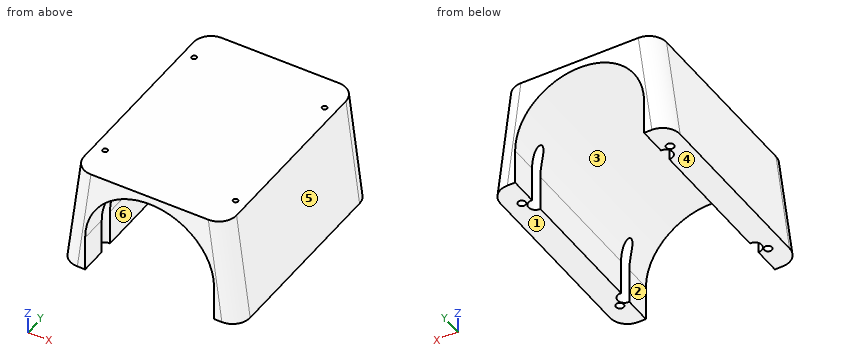
```python
from build123d import *

# Parameters (mm, degrees)
POCKET_DEPTH    = 110.201
SKETCH003_R     = 1.95
POCKET001_DEPTH = 30
SKETCH004_R     = 1.25
POCKET002_DEPTH = 55.001
SKETCH005_R     = 3.5
POCKET003_DEPTH = 50


with BuildPart() as part:
    # Sketch → Loft section 0
    with BuildSketch(Plane.XY):
        with BuildLine():
            Line((-37, 55.1), (37, 55.1))
            ThreePointArc((46, 46.1), (43.363961, 52.463961), (37, 55.1))
            Line((46, 46.1), (46, -46.1))
            ThreePointArc((37, -55.1), (43.363961, -52.463961), (46, -46.1))
            Line((37, -55.1), (-37, -55.1))
            ThreePointArc((-46, -46.1), (-43.363961, -52.463961), (-37, -55.1))
            Line((-46, -46.1), (-46, 46.1))
            ThreePointArc((-37, 55.1), (-43.363961, 52.463961), (-46, 46.1))
        make_face()
    # Sketch001 → Loft section 1
    with BuildSketch(Plane.XY.offset(55)):
        with BuildLine():
            Line((-30.05, 55.1), (30.05, 55.1))
            ThreePointArc((39.05, 46.1), (36.413961, 52.463961), (30.05, 55.1))
            Line((39.05, 46.1), (39.05, -46.1))
            ThreePointArc((30.05, -55.1), (36.413961, -52.463961), (39.05, -46.1))
            Line((30.05, -55.1), (-30.05, -55.1))
            ThreePointArc((-39.05, -46.1), (-36.413961, -52.463961), (-30.05, -55.1))
            Line((-39.05, -46.1), (-39.05, 46.1))
            ThreePointArc((-30.05, 55.1), (-36.413961, 52.463961), (-39.05, 46.1))
        make_face()
    loft()

    # Sketch002 (on Face5 of BaseFeature) → Pocket (cut, through all)
    with BuildSketch(Plane.XZ.offset(55.1)):
        with BuildLine():
            Line((33, 18), (33, 0))
            Line((33, 0), (-33, 0))
            Line((-33, 0), (-33, 18))
            ThreePointArc((33, 18), (0, 51), (-33, 18))
        make_face()
    extrude(amount=-POCKET_DEPTH, mode=Mode.SUBTRACT)

    # Sketch003 (on Face5 of Pocket) → Pocket001 (cut)
    with BuildSketch(Plane(origin=(0, 0, 0), x_dir=(1, 0, 0), z_dir=(0, 0, -1))):
        with Locations((-37.95, 41.3)):
            Circle(SKETCH003_R)
        with Locations((-37.95, -41.3)):
            Circle(SKETCH003_R)
        with Locations((37.95, -41.3)):
            Circle(SKETCH003_R)
        with Locations((37.95, 41.3)):
            Circle(SKETCH003_R)
    extrude(amount=-POCKET001_DEPTH, mode=Mode.SUBTRACT)

    # Sketch004 (on Face3 of Pocket001) → Pocket002 (cut, through all)
    with BuildSketch(Plane.XY.offset(55)):
        with Locations((-33.4, 37.35)):
            Circle(SKETCH004_R)
        with Locations((33.4, 37.35)):
            Circle(SKETCH004_R)
        with Locations((33.4, -37.65)):
            Circle(SKETCH004_R)
        with Locations((-33.4, -37.65)):
            Circle(SKETCH004_R)
    extrude(amount=-POCKET002_DEPTH, mode=Mode.SUBTRACT)

    # Sketch005 (on Face9 of Pocket002) → Pocket003 (cut)
    with BuildSketch(Plane(origin=(0, 0, 0), x_dir=(1, 0, 0), z_dir=(0, 0, -1))):
        with Locations((-33.4, -37.35)):
            Circle(SKETCH005_R)
        with Locations((33.4, -37.35)):
            Circle(SKETCH005_R)
        with Locations((-33.4, 37.65)):
            Circle(SKETCH005_R)
        with Locations((33.4, 37.65)):
            Circle(SKETCH005_R)
    extrude(amount=-POCKET003_DEPTH, mode=Mode.SUBTRACT)


solid = part.part
```
Verification items for the finished model (mm, model axes). Face numbers are marked on the shaded views. A direction names the side the tool comes from. Round coordinates to 2 decimals unless told otherwise and drop trailing zeros. Write each loop counter-clockwise with the first axis right and the second up, starting at its lowest first coordinate (ties: lowest second). Pieces come first, ordered by that corner, then holes. Notation, with made-up numbers: (43, 1.5) - (53, 1.5) arc R24 cw to (53, 28.5) - close; hole circle Ø3 at (19.25, 73.25). An arc over 180 degrees is marked (long way). Answer as a JSON object with one key per item and string values. Group by question number.
Q1. Section check B-B, the plane z = 37. Give the number of separate pieces and of enclosed holes in the cut face, plus the area to 3 significant figures.
Q2. Mould release check, pull along X, two halves, no side actions. Record for the marked faces 3, 4, 5 and 6: released by +X, released by -X, zero draft, split by the parting line, or undercut.
Q3. Go/stop test with flat-tipped pins: pin 1 Ø1.5 at (x, z) = (28.5, 31) entering from +Y; pin 2 Ø5 at (x, y) = (37.95, 41.3) entering from -Z; pin 3 Ø1 at (y, z) = (-32.5, 21.5) entering from -X; pin 4 Ø2.5 at (x, y) = (37.95, -41.3) entering from -Z. Record where each tip stops, or that it passes through.
Q4. Thickness scan on line 1 (Y direction, x = 33, z = 34.5); line 2 (X direction, y = -41.3, z = 21.5); line 3 (Y direction, x = -37, z = 10). Record the ranges inside material, lowest first.
Q5. Section check A-A, the plane y = -29. Enter the section's corners in (x, z), plus the area to 3 significant figures.
Q6. Tool access check on the marked faces 1 and 2. Record the directions out of +Z, -Z, +X, -X, +Y, -Y that give a thin tool (end or side, any length) a straight path to the whole face; none if there is none.
Found:
{
 "1": {"separate pieces": "2", "enclosed holes": "4", "area": "2,940 mm^2"},
 "2": {"face 3": "undercut", "face 4": "zero draft", "face 5": "released by +X", "face 6": "undercut"},
 "3": {"pin 1": "passes through", "pin 2": "stops at z = 0", "pin 3": "stops at x = -43.35", "pin 4": "stops at z = 30"},
 "4": {"line 1": "y = -55.09 to -41.13, -34.17 to 33.87, 40.83 to 55.09", "line 2": "x = -43.28 to -39.9, -36 to -32.81, 32.81 to 36, 39.9 to 43.28", "line 3": "y = -55.01 to -43, -39.6 to 39.6, 43 to 55.01"},
 "5": {"outline": "(-46, 0) - (-33, 0) - (-33, 18) arc R33 cw to (33, 18) - (33, 0) - (46, 0) - (39.05, 55) - (-39.05, 55) - close", "area": "1,780 mm^2"},
 "6": {"face 1": "-Z, +X, -X, +Y, -Y", "face 2": "-Z, +Y, -Y"}
}
